from build123d import *

# Parameters (mm, degrees)
SKETCH1_W                                       = 38
SKETCH1_H                                       = 20
BOSS_EXTRUDE1_DEPTH                             = 3
CSK_FOR_M3_FLAT_HEAD_MACHINE_SCREW1_D           = 3.3
CSK_FOR_M3_FLAT_HEAD_MACHINE_SCREW1_CSINK_D     = 6
CSK_FOR_M3_FLAT_HEAD_MACHINE_SCREW1_CSINK_ANGLE = 90


with BuildPart() as part:
    # Sketch1 → Boss-Extrude1 (new body)
    with BuildSketch(Plane.XY):
        with Locations((0, 10)):
            Rectangle(SKETCH1_W, SKETCH1_H)
    extrude(amount=BOSS_EXTRUDE1_DEPTH)

    # CSK for M3 Flat Head Machine Screw1 (through all)
    with Locations(Plane.XY.offset(3)):
        with Locations((-16, 16), (16, 16)):
            CounterSinkHole(CSK_FOR_M3_FLAT_HEAD_MACHINE_SCREW1_D / 2, CSK_FOR_M3_FLAT_HEAD_MACHINE_SCREW1_CSINK_D / 2, counter_sink_angle=CSK_FOR_M3_FLAT_HEAD_MACHINE_SCREW1_CSINK_ANGLE)


solid = part.part
Work out the finished part from the listing and answer in its coordinate system (mm). Round coordinates to 2 decimals unless told otherwise and drop trailing zeros. Order: outer loops, then holes, each group sorted by start corner. A loop starts at its lowest first (then second) coordinate and runs counter-clockwise, first axis right, second up. Notation, with made-up numbers: M -38.5,78 L 10.5,78 A15 cw 10.5,107 Z; hole C -22.5,82.5 d10. An arc over 180 degrees is marked long. One line per item, written item: value.
Q1. Straight lines are drawn through the part: line 1 (X direction, y = 16, z = 0.95); line 2 (Y direction, x = 16, z = 1.35); line 3 (Y direction, x = -15, z = 0.8). For each, find the intervals that lie inside material, in ascending order.
Derived:
line 1: -19 to -17.65, -14.35 to 14.35, 17.65 to 19
line 2: 0 to 14.35, 17.65 to 20
line 3: 0 to 14.69, 17.31 to 20
Q2. Determine the mould class of faces 1 (the face through (16, 18, 2)), 2 (the face through (-16, 18, 2)), 3 (the face through (19, 10, 1)), 4 (the face through (0, 0, 1)) for opening direction Y: released by +Y, released by -Y, zero draft, split by the parting line, or undercut.
Derived:
face 1: undercut
face 2: undercut
face 3: zero draft
face 4: released by -Y
Q3. Find section B-B on x = 16. Write down the section's boundary in (y, z).
Derived:
outline: M 0,0 L 14.35,0 L 14.35,1.65 L 13,3 L 0,3 Z; M 17.65,0 L 20,0 L 20,3 L 19,3 L 17.65,1.65 Z
Q4. Find section A-A on z = 2.5. Write down the section's boundary in (x, y).
Derived:
outline: M -19,0 L 19,0 L 19,20 L -19,20 Z; hole C -16,16 d5; hole C 16,16 d5
Q5. Find section C-C on z = 0.5. Write down the section's boundary in (x, y), then the cut area to 3 significant figures.
Derived:
outline: M -19,0 L 19,0 L 19,20 L -19,20 Z; hole C -16,16 d3.3; hole C 16,16 d3.3
area: 743 mm²
